Source: CAD feature listing. Evaluate the final solid. Frame: model axes, mm. Face numbers are marked on the shaded views. A direction names the side the tool comes from. Round coordinates to 2 decimals unless told otherwise and drop trailing zeros. Loops run counter-clockwise (first coordinate to the right, second up) from the corner with the lowest first, then second, coordinate; pieces in that order, holes last. Notation, with made-up numbers: M -17.75,73 L 18.25,73 A32 cw 18.25,110 Z; hole C 23.25,7 d7. An arc over 180 degrees is marked long. One line per item, written item: value.
from build123d import *

# Parameters (mm, degrees)
EXTRUSION1_DEPTH = 35


with BuildPart() as part:
    # Esquisse1 → Extrusion1 (new body)
    with BuildSketch(Plane.XY):
        with BuildLine():
            Line((4.7, -4.8), (4.7, 0))
            Line((4.7, 0), (5.8, 0))
            Line((5.8, 0), (5.8, -1.1))
            Line((5.8, -1.1), (5.25, -1.6))
            Line((5.25, -1.6), (5.8, -2.1))
            Line((5.8, -2.1), (5.8, -4.8))
            ThreePointArc((5.8, -4.8), (5.33137085, -5.93137085), (4.2, -6.4))
            Line((4.2, -6.4), (1.6, -6.4))
            ThreePointArc((1.6, -6.4), (0.46862915, -5.93137085), (0, -4.8))
            Line((0, -4.8), (0, -2.1))
            Line((0, -2.1), (0.55, -1.6))
            Line((0.55, -1.6), (0, -1.1))
            Line((0, -1.1), (0, 0))
            Line((0, 0), (1.1, 0))
            Line((1.1, 0), (1.1, -4.8))
            ThreePointArc((1.1, -4.8), (1.246446609, -5.153553391), (1.6, -5.3))
            Line((1.6, -5.3), (4.2, -5.3))
            ThreePointArc((4.2, -5.3), (4.553553391, -5.153553391), (4.7, -4.8))
        make_face()
    extrude(amount=EXTRUSION1_DEPTH)


solid = part.part
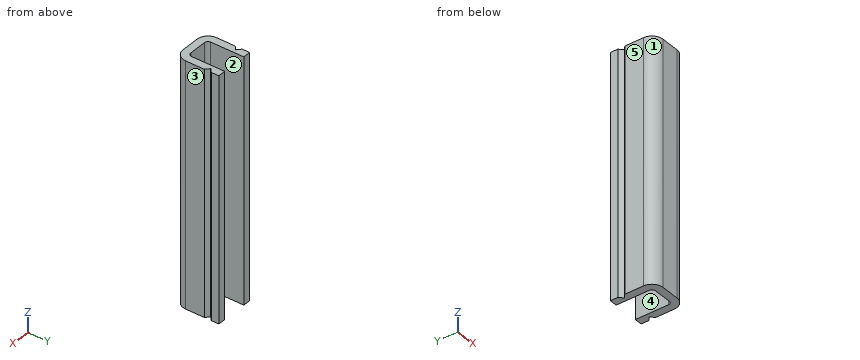
1. Pin query (flat end, axial travel): pin 1 (2 mm diameter, centred on x = 2.5, z = 19, fed in from +Y); pin 2 (1 mm diameter, centred on x = 4.5, y = -3.5, fed in from +Z). Return the tip coordinate at first contact, or that it passes through.
Report:
pin 1: stops at y = -5.29
pin 2: stops at z = 35
2. Section query C-C (x = 2.25). Return the cut outline in (y, z), and give its area (3 significant figures).
Report:
outline: M -6.4,0 L -5.3,0 L -5.3,35 L -6.4,35 Z
area: 38.5 mm2
3. Reachability of the marked faces 1 and 2 from +Z, -Z, +X, -X, +Y, -Y: full face, straight path, thin tool, end or side. Return the list, or none.
Report:
face 1: +Z, -Z, -X, -Y
face 2: +Z, -Z, +Y
4. Section query D-D (y = -6). Return the cut outline in (x, z).
Report:
outline: M 0.54,0 L 5.26,0 L 5.26,35 L 0.54,35 Z
5. Pull-direction query (X, two-part tool) for the marked faces 3, 4 and 5; classes: released by +X, released by -X, zero draft, split by the parting line, or undercut.
Report:
face 3: released by +X
face 4: undercut
face 5: released by -X
6. Ray query, line 1 (X direction, y = -2.5, z = 18.5); line 2 (Y direction, x = 3.75, z = 5); line 3 (X direction, y = -1.75, z = 16) (3 decimals). Return the intervals inside material, ascending. Write a range as [from, to].
Report:
line 1: x = [0, 1.1], [4.7, 5.8]
line 2: y = [-6.4, -5.3]
line 3: x = [0.385, 1.1], [4.7, 5.415]
7. Section query B-B (z = 4). Return the cut outline in (x, y).
Report:
outline: M 0,-4.8 A1.6 ccw 1.6,-6.4 L 4.2,-6.4 A1.6 ccw 5.8,-4.8 L 5.8,-2.1 L 5.25,-1.6 L 5.8,-1.1 L 5.8,0 L 4.7,0 L 4.7,-4.8 A0.5 cw 4.2,-5.3 L 1.6,-5.3 A0.5 cw 1.1,-4.8 L 1.1,0 L 0,0 L 0,-1.1 L 0.55,-1.6 L 0,-2.1 Z
8. Section query A-A (y = -2.75). Return the cut outline in (x, z), and give its area (3 significant figures).
Report:
outline: M 0,0 L 1.1,0 L 1.1,35 L 0,35 Z; M 4.7,0 L 5.8,0 L 5.8,35 L 4.7,35 Z
area: 77.0 mm2
